Answer from the drawing. Dimensions are ordinates in mm from the lowest x, y and z of the part. Give positions to 0.01 mm unless a question says otherwise; leave off trailing zeros. Write each loop counter-clockwise with the first axis right and the second up, starting at its lowest first coordinate (ties: lowest second). Pieces come first, ordered by that corner, then holes.
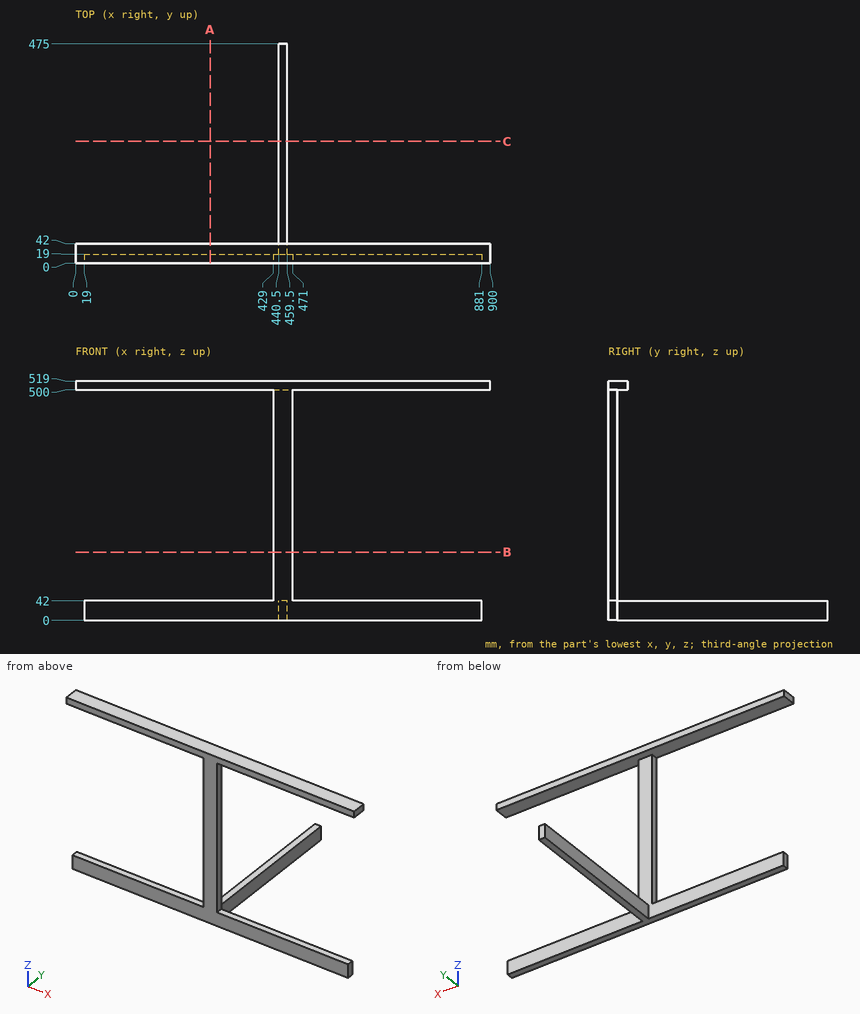
Item 1: Section A-A (x = 292) is taken. Write down the section's boundary in (y, z), and give its area (3 significant figures).
Result set:
outline: (0, 0) - (19, 0) - (19, 42) - (0, 42) - close; (0, 500) - (42, 500) - (42, 519) - (0, 519) - close
area: 1,600 mm2
Item 2: Section B-B (z = 148) is taken. Write down the section's boundary in (x, y), and give its area (3 significant figures).
Result set:
outline: (429, 0) - (471, 0) - (471, 19) - (429, 19) - close
area: 798 mm2
Item 3: Section C-C (y = 264) is taken. Write down the section's boundary in (x, z).
Result set:
outline: (440.5, 0) - (459.5, 0) - (459.5, 42) - (440.5, 42) - close
Item 4: Each of these flat-tipped pins is pushed along its axis until it touches: pin 1 Ø21 at (x, y) = (454.5, 220) entering from +Z; pin 2 Ø9.5 at (y, z) = (6.5, 28.5) entering from -X; pin 3 Ø5.5 at (y, z) = (7, 164) entering from -X. Where does it stop, or does it pass through?
Result set:
pin 1: stops at z = 42
pin 2: stops at x = 19
pin 3: stops at x = 429
Item 5: Find the intervals of material crossed by line 1 along Z through (x, y) = (554, 24), in increasing order.
Result set:
line 1: z = 500 to 519
